```python
from build123d import *

# Parameters (mm, degrees)
F0_W      = 69
F0_H      = 40
F1_DEPTH  = 18
F2_W      = 11
F2_H      = 32
F3_DEPTH  = 36.001
F4_W      = 22
F4_H      = 24
F5_DEPTH  = 36.001
F6_R      = 12
F7_DEPTH  = 36.001
F8_W      = 16
F8_H      = 16
F9_DEPTH  = 58.001
F10_W     = 24
F10_H     = 4
F11_DEPTH = 8.001


with BuildPart() as f1:
    # F0 (on Right) → F1 (new body, symmetric)
    with BuildSketch(Plane.YZ):
        with Locations((-5.739541, 0)):
            Rectangle(F0_W, F0_H)
    extrude(amount=F1_DEPTH, both=True)

    # F2 (on face) → F3 (cut, through all)
    with BuildSketch(Plane.YZ.offset(18)):
        with Locations((-34.739541, 4)):
            Rectangle(F2_W, F2_H)
    extrude(amount=-F3_DEPTH, mode=Mode.SUBTRACT)

    # F4 (on face) → F5 (cut, through all)
    with BuildSketch(Plane.YZ.offset(18)):
        with Locations((17.760459, 0)):
            Rectangle(F4_W, F4_H)
    extrude(amount=-F5_DEPTH, mode=Mode.SUBTRACT)

    # F6 (on face) → F7 (cut, through all)
    with BuildSketch(Plane.YZ.offset(18)):
        with Locations((-11.239541, 0)):
            Circle(F6_R)
    extrude(amount=-F7_DEPTH, mode=Mode.SUBTRACT)

    # F8 (on face) → F9 (cut, through all)
    with BuildSketch(Plane.XZ.offset(29.239541)):
        Rectangle(F8_W, F8_H)
    extrude(amount=-F9_DEPTH, mode=Mode.SUBTRACT)

    # F10 (on face) → F11 (cut, through all)
    with BuildSketch(Plane.XY.offset(-12)):
        with Locations((0, -38.239541)):
            Rectangle(F10_W, F10_H)
    extrude(amount=-F11_DEPTH, mode=Mode.SUBTRACT)


solid = f1.part
```
The listing builds one solid part. Answer for the finished solid, in the listing's coordinates (mm). A direction names the side the tool comes from. Coordinates: 2 decimals unless noted, no trailing zeros. Write each loop counter-clockwise with the first axis right and the second up, starting at its lowest first coordinate (ties: lowest second). Pieces come first, ordered by that corner, then holes. Notation, with made-up numbers: (-15.75, 28) - (27.25, 28) arc R15 ccw to (27.25, 38) - close; hole circle Ø4 at (48, 88.5). An arc over 180 degrees is marked (long way). Return JSON: item names as keys, results as strings. Group by question number.
Q1. Flat-ended cylindrical pins translate along their axes: pin 1 Ø4 at (x, z) = (1, -15) entering from -Y; pin 2 Ø4 at (x, z) = (-7.5, 0.5) entering from -Y; pin 3 Ø7 at (x, z) = (-8, -5.5) entering from +Y. Find the tip coordinate at first contact, or state that the pin passes through.
Q2. For a pull along Y with two mould halves and no side action, classify faces 1 (the cylindrical face through (0.3, -12.8, 11.9)), 2 (the flat face through (0, -25, -8)), 3 (the flat face through (15, -40.24, -16)), 4 (the flat face through (8.3, 6.76, -0.2)) as +Y half, -Y half, draft (parallel to the pull), parting line (faces both ways), or undercut.
Q3. Find the intervals of material crossed by line 1 along Z through (x, y) = (-3, 24); line 2 along X through (y, z) = (-26, -6.5); line 3 along Y through (x, z) = (10, 0), in increasing order. Write a range as [from, to].
Q4. The part is cut by section D-D on z = 11. Write down the section's boundary in (x, y), and give its area (3 significant figures).
Q5. The part is cut by section C-C on z = 0. Write down the section's boundary in (x, y).
Q6. The part is cut by section B-B on x = 4. Write down the section's boundary in (y, z), and give its area (3 significant figures).
Q7. The part is cut by section A-A on y = 21.5. Write down the section's boundary in (x, z).
Q8. Which of the six approach directions +Z, -Z, +X, -X, +Y, -Y give full straight-line access (tool end or side, diameter ignored) to faces 5 (the flat face through (-8, -26, 0)), 6 (the flat face through (-12, -38, -16)), 7 (the flat face through (0, -29.24, 11)), 8 (the flat face through (0, 18, 12))?
Evaluation:
{
 "1": {"pin 1": "stops at y = -36.24", "pin 2": "stops at y = -29.24", "pin 3": "stops at y = 6.76"},
 "2": {"face 1": "undercut", "face 2": "draft", "face 3": "-Y half", "face 4": "+Y half"},
 "3": {"line 1": "z = [-20, -12], [12, 20]", "line 2": "x = [-18, -8], [8, 18]", "line 3": "y = [-29.24, -23.24], [0.76, 6.76]"},
 "4": {"outline": "(-18, -29.24) - (18, -29.24) - (18, -16.04) - (-18, -16.04) - close; (-18, -6.44) - (18, -6.44) - (18, 6.76) - (-18, 6.76) - close", "area": "951 mm2"},
 "5": {"outline": "(-18, -29.24) - (-8, -29.24) - (-8, -23.24) - (-18, -23.24) - close; (-18, 0.76) - (-8, 0.76) - (-8, 6.76) - (-18, 6.76) - close; (8, -29.24) - (18, -29.24) - (18, -23.24) - (8, -23.24) - close; (8, 0.76) - (18, 0.76) - (18, 6.76) - (8, 6.76) - close"},
 "6": {"outline": "(-36.24, -20) - (28.76, -20) - (28.76, -12) - (6.76, -12) - (6.76, -8) - (-2.3, -8) arc R12 cw to (-20.18, -8) - (-29.24, -8) - (-29.24, -12) - (-36.24, -12) - close; (-29.24, 8) - (-20.18, 8) arc R12 cw to (-2.3, 8) - (6.76, 8) - (6.76, 12) - (28.76, 12) - (28.76, 20) - (-29.24, 20) - close", "area": "1,170 mm2"},
 "7": {"outline": "(-18, -20) - (18, -20) - (18, -12) - (-18, -12) - close; (-18, 12) - (18, 12) - (18, 20) - (-18, 20) - close"},
 "8": {"face 5": "+Y, -Y", "face 6": "+Z, -Z, -Y", "face 7": "+Z, +X, -X, -Y", "face 8": "+X, -X, +Y"}
}
